from build123d import *

# Parameters (mm, degrees)
BOSS_EXTRUDE1_DEPTH   = 3
BOSS_EXTRUDE2_DEPTH   = 24
SKETCH3_W             = 1.3
SKETCH3_H             = 10.4
BOSS_EXTRUDE3_DEPTH   = 16.5
M5X0_8_TAPPED_HOLE1_D = 4.2
M5X0_8_TAPPED_HOLE2_D = 4.2


with BuildPart() as part:
    # Sketch1 → Boss-Extrude1 (new body, symmetric)
    with BuildSketch(Plane.XY):
        with BuildLine():
            Line((0, 26), (0, 0))
            Line((0, 0), (25.5, 0))
            Line((25.5, 0), (25.5, 5))
            Line((25.5, 5), (8, 5))
            ThreePointArc((8, 5), (5.878679656, 5.878679656), (5, 8))
            Line((5, 8), (5, 26))
            Line((5, 26), (0, 26))
        make_face()
    extrude(amount=BOSS_EXTRUDE1_DEPTH, both=True)

    # Sketch2 → Boss-Extrude2 (add)
    with BuildSketch(Plane(origin=(25.5, 0, 0), x_dir=(0, 0, -1), z_dir=(1, 0, 0))):
        Polygon((-3, 0), (-5, 3.75), (5, 3.75), (3, 0), align=None)
    extrude(amount=-BOSS_EXTRUDE2_DEPTH)

    # Sketch3 → Boss-Extrude3 (add)
    with BuildSketch(Plane(origin=(0, 26, 0), x_dir=(1, 0, 0), z_dir=(0, 1, 0))):
        with Locations((2.15, 0)):
            Rectangle(SKETCH3_W, SKETCH3_H)
    extrude(amount=-BOSS_EXTRUDE3_DEPTH)

    # M5x0.8 Tapped Hole1 (through all)
    with Locations(Plane(origin=(0, 5, 0), x_dir=(1, 0, 0), z_dir=(0, 1, 0))):
        with Locations((18.5, 0)):
            Hole(M5X0_8_TAPPED_HOLE1_D / 2)

    # M5x0.8 Tapped Hole2 (through all)
    with Locations(Plane(origin=(5, 0, 0), x_dir=(0, 0, -1), z_dir=(1, 0, 0))):
        with Locations((0, 20.2)):
            Hole(M5X0_8_TAPPED_HOLE2_D / 2)


solid = part.part
Source: CAD feature listing. Evaluate the final solid. Frame: model axes, mm. A direction names the side the tool comes from. Give positions to 0.01 mm unless a question says otherwise; leave off trailing zeros. Loops run counter-clockwise (first coordinate to the right, second up) from the corner with the lowest first, then second, coordinate; pieces in that order, holes last. Notation, with made-up numbers: (-16.5, 77.25) -> (-9.5, 77.25) arc R24 ccw to (-9.5, 110.25) -> close; hole circle Ø1 at (19, 22). An arc over 180 degrees is marked (long way). Use a Markdown table: item, result. Add a question column.
1) Pull-direction query (Y, two-part tool) for faces 1 (the face through (1.5, 2.3, 3.8)), 2 (the face through (2, 9.5, 4)), 3 (the face through (15, 5, 0)); classes: +Y half, -Y half, draft (parallel to the pull), parting line (faces both ways), or undercut.
2) First-contact query: pin 1 (0.6 mm diameter, centred on x = 2.5, z = -4, fed in from -Y); pin 2 (1.8 mm diameter, centred on y = 14.5, z = 4.5, fed in from -X); pin 3 (1 mm diameter, centred on x = 13.5, z = 4, fed in from +Y); pin 4 (3 mm diameter, centred on x = 6.5, z = -0.5, fed in from -Y). Flat tips, straight axial feed; report the tip coordinate or a pass-through.
3) Section query B-B, the plane x = 18.5. Return the cut outline in (y, z).
4) Line query: line 1 along Y through (x, z) = (3.8, 0); line 2 along Y through (x, z) = (10.25, 2). Output: solid intervals per line, ascending. Write a range as [from, to].
5) Section query C-C, the plane y = 20.2. Return the cut outline in (x, z).
6) Section query A-A, the plane z = 0. Return the cut outline in (x, y), then the cut area to 3 significant figures.
7) Reachability of faces 4 (the face through (2.8, 18, -4)), 5 (the face through (5, 17, 0)), 6 (the face through (1.5, 18, 4)) from +Z, -Z, +X, -X, +Y, -Y: full face, straight path, thin tool, end or side. Return the list, or none.
8) Section query D-D, the plane x = 15.25. Return the cut outline in (y, z), then the cut area to 3 significant figures.
Numbers:
| question | item | result |
|---|---|---|
| 1 | face 1 | draft |
| 1 | face 2 | undercut |
| 1 | face 3 | +Y half |
| 2 | pin 1 | stops at y = 1.31 |
| 2 | pin 2 | stops at x = 1.5 |
| 2 | pin 3 | stops at y = 3.75 |
| 2 | pin 4 | stops at y = 0 |
| 3 | outline | (0, -3) -> (3.75, -5) -> (3.75, -3) -> (5, -3) -> (5, -2.1) -> (0, -2.1) -> close; (0, 2.1) -> (5, 2.1) -> (5, 3) -> (3.75, 3) -> (3.75, 5) -> (0, 3) -> close |
| 4 | line 1 | y = [0, 18.1], [22.3, 26] |
| 4 | line 2 | y = [0, 5] |
| 5 | outline | (0, -3) -> (1.5, -3) -> (1.5, -5.2) -> (2.8, -5.2) -> (2.8, -3) -> (5, -3) -> (5, -2.1) -> (0, -2.1) -> close; (0, 2.1) -> (5, 2.1) -> (5, 3) -> (2.8, 3) -> (2.8, 5.2) -> (1.5, 5.2) -> (1.5, 3) -> (0, 3) -> close |
| 6 | outline | (0, 0) -> (16.4, 0) -> (16.4, 5) -> (8, 5) arc R3 cw to (5, 8) -> (5, 18.1) -> (0, 18.1) -> close; (0, 22.3) -> (5, 22.3) -> (5, 26) -> (0, 26) -> close; (20.6, 0) -> (25.5, 0) -> (25.5, 5) -> (20.6, 5) -> close |
| 6 | area | 192 mm2 |
| 7 | face 4 | -Z, +X, +Y |
| 7 | face 5 | +Z, -Z, +X, +Y |
| 7 | face 6 | +Z, -X, +Y, -Y |
| 8 | outline | (0, -3) -> (3.75, -5) -> (3.75, -3) -> (5, -3) -> (5, 3) -> (3.75, 3) -> (3.75, 5) -> (0, 3) -> close |
| 8 | area | 37.5 mm2 |
